Design review of the part shown in the three views and the two pictorial views. Dimensions are in mm from the part's minimum x, y and z. Coordinates: 2 decimals unless noted, no trailing zeros. Write each loop counter-clockwise with the first axis right and the second up, starting at its lowest first coordinate (ties: lowest second). Pieces come first, ordered by that corner, then holes. Notation, with made-up numbers: (42.5, 57.5) -> (60.5, 57.5) arc R9 cw to (60.5, 70.5) -> close; hole circle Ø4 at (58, 86). An arc over 180 degrees is marked (long way). Answer in a Markdown table with one row per item. Add a question column.
Item 1: Take a section at A-A, the plane y = 73. Write out the cut boundary in (x, z) (1 decimal), and give its area (3 significant figures).
Item 2: Take a section at C-C, the plane x = 162. Write out the cut boundary in (y, z).
Item 3: Take a section at B-B, the plane z = 70. Write out the cut boundary in (x, y) (1 decimal), and give its area (4 significant figures).
Item 4: Take a section at D-D, the plane x = 35. Write out the cut boundary in (y, z).
Item 5: Draft analysis for pull direction X (two halves, no side actions). For the marked faces 1, 2, 3 and 4, state which applies: released by +X, released by -X, zero draft, split by the parting line, or undercut.
Item 6: Clearance check with flat-ended pins moving along their axes: P1, Ø9, axis at x = 125, z = 72, coming from the +Y side; P2, Ø17, axis at x = 225.77, z = 15, coming from the +Y side; P3, Ø9, axis at x = 225.77, z = 15, coming from the +Y side. State where each tip first meets the part, or that it passes through.
Item 7: To check wall thickness, follow line 1 (Z direction, x = 15, y = 69); line 2 (Z direction, x = 127, y = 56); line 3 (X direction, y = 81.25, z = 15) (1 decimal). State the ranges of each line that lie inside material, in increasing order.
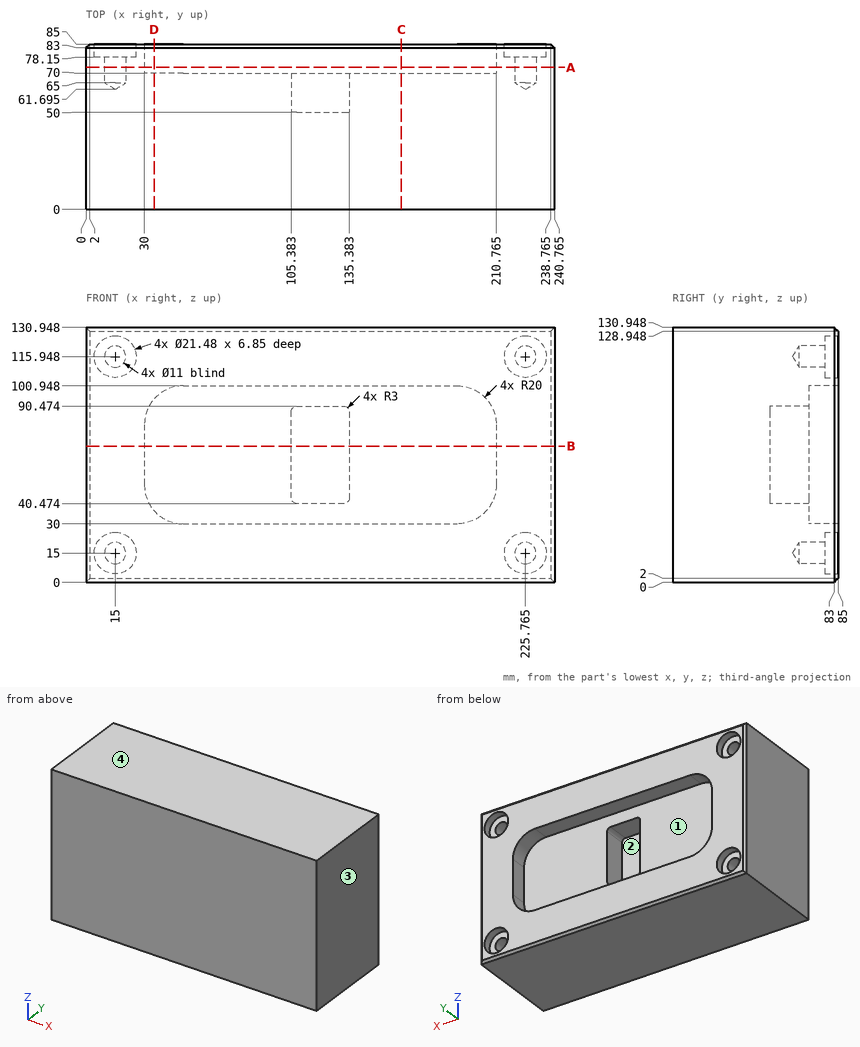
Answers:
| question | item | result |
|---|---|---|
| 1 | outline | (0, 0) -> (240.8, 0) -> (240.8, 130.9) -> (0, 130.9) -> close; hole circle Ø11 at (15, 15); hole circle Ø11 at (15, 115.9); hole (30, 50) arc R20 ccw to (50, 30) -> (190.8, 30) arc R20 ccw to (210.8, 50) -> (210.8, 80.9) arc R20 ccw to (190.8, 100.9) -> (50, 100.9) arc R20 ccw to (30, 80.9) -> close; hole circle Ø11 at (225.8, 15); hole circle Ø11 at (225.8, 115.9) |
| 1 | area | 18,700 mm^2 |
| 2 | outline | (0, 0) -> (83, 0) -> (85, 2) -> (85, 30) -> (70, 30) -> (70, 100.95) -> (85, 100.95) -> (85, 128.95) -> (83, 130.95) -> (0, 130.95) -> close |
| 3 | outline | (0, 0) -> (240.8, 0) -> (240.8, 83) -> (238.8, 85) -> (210.8, 85) -> (210.8, 70) -> (135.4, 70) -> (135.4, 50) -> (105.4, 50) -> (105.4, 70) -> (30, 70) -> (30, 85) -> (2, 85) -> (0, 83) -> close |
| 3 | area | 17,150 mm^2 |
| 4 | outline | (0, 0) -> (83, 0) -> (85, 2) -> (85, 36.77) -> (70, 36.77) -> (70, 94.18) -> (85, 94.18) -> (85, 128.95) -> (83, 130.95) -> (0, 130.95) -> close |
| 5 | face 1 | undercut |
| 5 | face 2 | undercut |
| 5 | face 3 | released by +X |
| 5 | face 4 | zero draft |
| 6 | P1 | stops at y = 50 |
| 6 | P2 | stops at y = 78.15 |
| 6 | P3 | stops at y = 64.4 |
| 7 | line 1 | z = 0 to 9.5, 20.5 to 110.45, 121.45 to 130.95 |
| 7 | line 2 | z = 0 to 40.47, 90.47 to 130.95 |
| 7 | line 3 | x = 0 to 4.3, 25.7 to 215, 236.5 to 240.8 |
